from build123d import *

# Parameters (mm, degrees)
SKETCH1_W           = 95
SKETCH1_H           = 95
BOSS_EXTRUDE1_DEPTH = 25
SKETCH2_R           = 7.75
CUT_EXTRUDE2_DEPTH  = 100
SKETCH3_R           = 17
CUT_EXTRUDE3_DEPTH  = 22
CUT_EXTRUDE4_START  = -22
SKETCH4_R           = 17
CUT_EXTRUDE4_DEPTH  = 22
SKETCH5_W           = 6.246993927
SKETCH5_H           = 25
CUT_EXTRUDE5_DEPTH  = 22
SKETCH6_W           = 7.178723585
SKETCH6_H           = 25
CUT_EXTRUDE6_DEPTH  = 22
SKETCH8_W           = 99.503929421
SKETCH8_H           = 3.5
CUT_EXTRUDE7_DEPTH  = 100
SKETCH9_W           = 8.3
SKETCH9_H           = 15.5
CUT_EXTRUDE11_DEPTH = 100
SKETCH13_W          = 87
SKETCH13_H          = 15.5
CUT_EXTRUDE12_DEPTH = 2
SKETCH14_W          = 25.5
SKETCH14_H          = 47
CUT_EXTRUDE14_DEPTH = 18.5
SKETCH16_W          = 24.75
SKETCH16_H          = 47
CUT_EXTRUDE15_DEPTH = 5
SKETCH17_W          = 20.919567191
SKETCH17_H          = 47
CUT_EXTRUDE16_DEPTH = 5
CUT_EXTRUDE17_DEPTH = 100
FILLET6_R           = 1.5
FILLET7_R           = 1.5
FILLET8_R           = 1.5
FILLET9_R           = 1.5
SKETCH19_W          = 12.12120401
SKETCH19_H          = 21.5
CUT_EXTRUDE20_DEPTH = 100
SKETCH20_W          = 5.709228799
SKETCH20_H          = 91
CUT_EXTRUDE23_DEPTH = 100
SKETCH21_W          = 6
SKETCH21_H          = 47
CUT_EXTRUDE26_DEPTH = 40
CHAMFER1_SIZE       = 2
SKETCH22_W          = 15
SKETCH22_H          = 10
CUT_EXTRUDE27_DEPTH = 4
SKETCH23_W          = 2
SKETCH23_H          = 10
CUT_EXTRUDE28_DEPTH = 54
CHAMFER2_SIZE       = 2
CHAMFER3_SIZE       = 4
CHAMFER4_SIZE       = 4
CUT_EXTRUDE29_DEPTH = 100


with BuildPart() as part:
    # Sketch1 → Boss-Extrude1 (new body)
    with BuildSketch(Plane(origin=(0, 0, 0), x_dir=(1, 0, 0), z_dir=(0, 1, 0))):
        with Locations((3.271948822, -17.506298191)):
            Rectangle(SKETCH1_W, SKETCH1_H)
    extrude(amount=BOSS_EXTRUDE1_DEPTH)

    # Sketch2 → Cut-Extrude2 (cut)
    with BuildSketch(Plane.XY.offset(65.006298191)):
        with Locations((-29.228051178, 10.75)):
            Circle(SKETCH2_R)
        with Locations((15.771948822, 10.75)):
            Circle(SKETCH2_R)
    extrude(amount=-CUT_EXTRUDE2_DEPTH, mode=Mode.SUBTRACT)

    # Sketch3 → Cut-Extrude3 (cut)
    with BuildSketch(Plane.XY.offset(65.006298191)):
        with Locations((-29.228051178, 10.75)):
            Circle(SKETCH3_R)
        with Locations((15.771948822, 10.75)):
            Circle(SKETCH3_R)
    extrude(amount=-CUT_EXTRUDE3_DEPTH, mode=Mode.SUBTRACT)

    # Sketch4 → Cut-Extrude4 (cut)
    with BuildSketch(Plane(origin=(0, 0, -29.993701809), x_dir=(-1, 0, 0), z_dir=(0, 0, -1)).offset(CUT_EXTRUDE4_START)):
        with Locations((-15.771948822, 10.75)):
            Circle(SKETCH4_R)
        with Locations((29.228051178, 10.75)):
            Circle(SKETCH4_R)
    extrude(amount=CUT_EXTRUDE4_DEPTH, mode=Mode.SUBTRACT)

    # Sketch5 → Cut-Extrude5 (cut)
    with BuildSketch(Plane.XY.offset(65.006298191)):
        with Locations((-41.104554214, 12.5)):
            Rectangle(SKETCH5_W, SKETCH5_H)
    extrude(amount=-CUT_EXTRUDE5_DEPTH, mode=Mode.SUBTRACT)

    # Sketch6 → Cut-Extrude6 (cut)
    with BuildSketch(Plane(origin=(0, 0, -29.993701809), x_dir=(-1, 0, 0), z_dir=(0, 0, -1))):
        with Locations((40.638689386, 12.5)):
            Rectangle(SKETCH6_W, SKETCH6_H)
    extrude(amount=-CUT_EXTRUDE6_DEPTH, mode=Mode.SUBTRACT)

    # Sketch8 → Cut-Extrude7 (cut)
    with BuildSketch(Plane(origin=(0, 0, -29.993701809), x_dir=(-1, 0, 0), z_dir=(0, 0, -1))):
        with Locations((-1.019984112, 23.25)):
            Rectangle(SKETCH8_W, SKETCH8_H)
    extrude(amount=-CUT_EXTRUDE7_DEPTH, mode=Mode.SUBTRACT)

    # Sketch9 → Cut-Extrude11 (cut)
    with BuildSketch(Plane.XY.offset(65.006298191)):
        with Locations((-7.828051178, 10.75)):
            Rectangle(SKETCH9_W, SKETCH9_H)
    extrude(amount=-CUT_EXTRUDE11_DEPTH, mode=Mode.SUBTRACT)

    # Sketch13 → Cut-Extrude12 (cut)
    with BuildSketch(Plane.ZY.offset(3.678051178)):
        with Locations((17.506298191, 10.75)):
            Rectangle(SKETCH13_W, SKETCH13_H)
    extrude(amount=-CUT_EXTRUDE12_DEPTH, mode=Mode.SUBTRACT)

    # Sketch14 → Cut-Extrude14 (cut)
    with BuildSketch(Plane(origin=(0, 21.5, 0), x_dir=(1, 0, 0), z_dir=(0, 1, 0))):
        with Locations((-6.728051178, -17.506298191)):
            Rectangle(SKETCH14_W, SKETCH14_H)
    extrude(amount=-CUT_EXTRUDE14_DEPTH, mode=Mode.SUBTRACT)

    # Sketch16 → Cut-Extrude15 (cut)
    with BuildSketch(Plane(origin=(0, 21.5, 0), x_dir=(1, 0, 0), z_dir=(0, 1, 0))):
        with Locations((-29.853051178, -17.506298191)):
            Rectangle(SKETCH16_W, SKETCH16_H)
    extrude(amount=-CUT_EXTRUDE15_DEPTH, mode=Mode.SUBTRACT)

    # Sketch17 → Cut-Extrude16 (cut)
    with BuildSketch(Plane(origin=(0, 21.5, 0), x_dir=(1, 0, 0), z_dir=(0, 1, 0))):
        with Locations((16.481732418, -17.506298191)):
            Rectangle(SKETCH17_W, SKETCH17_H)
    extrude(amount=-CUT_EXTRUDE16_DEPTH, mode=Mode.SUBTRACT)

    # Sketch18 → Cut-Extrude17 (cut)
    with BuildSketch(Plane.XY.offset(65.006298191)):
        with BuildLine():
            Line((34.66639245, 12.75), (37.680851122, 12.75))
            ThreePointArc((37.680851122, 12.75), (37.300376381, 15.28065192), (36.628602437, 17.75))
            Line((36.628602437, 17.75), (33.435470555, 17.75))
            ThreePointArc((33.435470555, 17.75), (34.221100776, 15.291893017), (34.66639245, 12.75))
        make_face()
        with BuildLine():
            Line((34.66639245, 8.75), (37.680851122, 8.75))
            ThreePointArc((37.680851122, 8.75), (37.300376381, 6.21934808), (36.628602437, 3.75))
            Line((36.628602437, 3.75), (33.435470555, 3.75))
            ThreePointArc((33.435470555, 3.75), (34.221100776, 6.208106983), (34.66639245, 8.75))
        make_face()
    extrude(amount=-CUT_EXTRUDE17_DEPTH, mode=Mode.SUBTRACT)

    # Fillet6
    fillet6_edges = [part.edges().sort_by_distance(p)[0] for p in [
        (33.435470555, 17.75, 17.506298191),
        (36.628602437, 17.75, 17.506298191),
    ]]
    fillet(fillet6_edges, radius=FILLET6_R - 0.0001)  # a hair under: the kernel refuses the full size

    # Fillet7
    fillet7_edges = [part.edges().sort_by_distance(p)[0] for p in [
        (37.680851122, 12.75, 17.506298191),
        (34.66639245, 12.75, 17.506298191),
    ]]
    fillet(fillet7_edges, radius=FILLET7_R - 0.0001)  # a hair under: the kernel refuses the full size

    # Fillet8
    fillet8_edges = [part.edges().sort_by_distance(p)[0] for p in [
        (33.435470555, 3.75, 17.506298191),
        (36.628602437, 3.75, 17.506298191),
    ]]
    fillet(fillet8_edges, radius=FILLET8_R - 0.0001)  # a hair under: the kernel refuses the full size

    # Fillet9
    fillet9_edges = [part.edges().sort_by_distance(p)[0] for p in [
        (37.680851122, 8.75, 17.506298191),
        (34.66639245, 8.75, 17.506298191),
    ]]
    fillet(fillet9_edges, radius=FILLET9_R - 0.0001)  # a hair under: the kernel refuses the full size

    # Sketch19 → Cut-Extrude20 (cut)
    with BuildSketch(Plane.XY.offset(65.006298191)):
        with Locations((44.711346817, 10.75)):
            Rectangle(SKETCH19_W, SKETCH19_H)
    extrude(amount=-CUT_EXTRUDE20_DEPTH, mode=Mode.SUBTRACT)

    # Sketch20 → Cut-Extrude23 (cut)
    with BuildSketch(Plane(origin=(0, 21.5, 0), x_dir=(1, 0, 0), z_dir=(0, 1, 0))):
        with Locations((35.796130413, -17.506298191)):
            Rectangle(SKETCH20_W, SKETCH20_H)
    extrude(amount=-CUT_EXTRUDE23_DEPTH, mode=Mode.SUBTRACT)

    # Sketch21 → Cut-Extrude26 (cut)
    with BuildSketch(Plane(origin=(0, 21.5, 0), x_dir=(1, 0, 0), z_dir=(0, 1, 0))):
        with Locations((29.941516013, -17.506298191)):
            Rectangle(SKETCH21_W, SKETCH21_H)
    extrude(amount=-CUT_EXTRUDE26_DEPTH, mode=Mode.SUBTRACT)

    # Chamfer1
    chamfer1_edges = [part.edges().sort_by_distance(p)[0] for p in [
        (26.941516013, 16.5, 17.506298191),
    ]]
    chamfer(chamfer1_edges, length=CHAMFER1_SIZE)

    # Sketch22 → Cut-Extrude27 (cut)
    with BuildSketch(Plane(origin=(0, 0, 0), x_dir=(-1, 0, 0), z_dir=(0, -1, 0))):
        with Locations((34.728051178, -17.506298191)):
            Rectangle(SKETCH22_W, SKETCH22_H)
    extrude(amount=-CUT_EXTRUDE27_DEPTH, mode=Mode.SUBTRACT)

    # Sketch23 → Cut-Extrude28 (cut)
    with BuildSketch(Plane(origin=(0, 0, 0), x_dir=(-1, 0, 0), z_dir=(0, -1, 0))):
        with Locations((43.228051178, -17.506298191)):
            Rectangle(SKETCH23_W, SKETCH23_H)
    extrude(amount=-CUT_EXTRUDE28_DEPTH, mode=Mode.SUBTRACT)

    # Chamfer2
    chamfer2_edges = [part.edges().sort_by_distance(p)[0] for p in [
        (-42.228051178, 4, 17.506298191),
    ]]
    chamfer(chamfer2_edges, length=CHAMFER2_SIZE)

    # Chamfer3
    chamfer3_edges = [part.edges().sort_by_distance(p)[0] for p in [
        (-44.228051178, 0, 2.256298191),
    ]]
    chamfer(chamfer3_edges, length=CHAMFER3_SIZE)

    # Chamfer4
    chamfer4_edges = [part.edges().sort_by_distance(p)[0] for p in [
        (-44.228051178, 0, 32.756298191),
    ]]
    chamfer(chamfer4_edges, length=CHAMFER4_SIZE)

    # Sketch24 → Cut-Extrude29 (cut)
    with BuildSketch(Plane.XY.offset(65.006298191)):
        with BuildLine():
            Line((36.983688261, 16.579680704), (37.862836804, 12.677489289))
            ThreePointArc((37.862836804, 12.677489289), (36.729195727, 10.884486805), (34.936193243, 12.018127881))
            Line((34.936193243, 12.018127881), (34.0570447, 15.920319296))
            ThreePointArc((34.0570447, 15.920319296), (35.190685776, 17.713321781), (36.983688261, 16.579680704))
        make_face()
        with BuildLine():
            Line((37.434280479, 6.920319296), (36.555131936, 3.018127881))
            ThreePointArc((36.555131936, 3.018127881), (34.762129451, 1.884486805), (33.628488375, 3.677489289))
            Line((33.628488375, 3.677489289), (34.507636918, 7.579680704))
            ThreePointArc((34.507636918, 7.579680704), (36.300639403, 8.713321781), (37.434280479, 6.920319296))
        make_face()
    extrude(amount=-CUT_EXTRUDE29_DEPTH, mode=Mode.SUBTRACT)


solid = part.part
Can you work these out from the model? Positions are in its coordinate system, mm. A direction names the side the tool comes from. Coordinates: 2 decimals unless noted, no trailing zeros. Order: outer loops, then holes, each group sorted by start corner. A loop starts at its lowest first (then second) coordinate and runs counter-clockwise, first axis right, second up. Notation, with made-up numbers: M -12.75,59 L 33.25,59 A20 ccw 33.25,82 Z; hole C 42.5,35 d11. An arc over 180 degrees is marked long. Answer as CSV lines item,"result".
(1) Suppose I cut it at C-C on x = 30. Please give me the cut outline in (y, z).
Geometry check:
outline,"M 0,-29.99 L 1.45,-29.99 L 1.45,-7.99 L 20.05,-7.99 L 20.05,-29.99 L 21.5,-29.99 L 21.5,-5.99 L 0,-5.99 Z; M 0,41.01 L 21.5,41.01 L 21.5,65.01 L 20.05,65.01 L 20.05,43.01 L 1.45,43.01 L 1.45,65.01 L 0,65.01 Z"
(2) Suppose I cut it at A-A on z = 56. Please give me the cut outline in (x, y), plus the area to 3 significant figures.
Geometry check:
outline,"M -16.06,0 L 2.6,0 A17 cw 2.6,21.5 L -16.06,21.5 A17 cw Z; M 28.94,0 L 32.94,0 L 32.94,21.5 L 28.94,21.5 A17 cw Z; hole M -11.98,3 L -1.68,3 L -1.68,18.5 L -11.98,18.5 Z"
area,"159 mm^2"
(3) On a 3-axis mill with a long thin cutter (end or side, diameter ignored), from which of +Z, -Z, +X, -X, +Y, -Y can I reach the whole of each face in a straight line? I mean faces 1 (the flat face through (34.28, 6.57, -28.98)), 2 (the flat face through (24, 11, -7.994)), 3 (the cylindrical face through (-1.227, 10.913, 54.16)), 4 (the flat face through (32.942, 11, 52)). Say none if no direction works.
Geometry check:
face 1,"+Z, -Z"
face 2,"-Z"
face 3,"+Z"
face 4,"+X, +Y, -Y"
(4) Please list where these lines run through material, in increasing order: L1, parallel to Z at x = 19.5, y = 20.5; L2, parallel to Y at x = -3.5, z = 51.5; L3, parallel to X at y = 9.75, z = -7.5.
Geometry check:
L1,"-7.99 to -5.99, 41.01 to 43.01"
L2,"0 to 3, 18.5 to 21.5"
L3,"-44.23 to -36.91, -21.54 to -11.98, -1.68 to 8.09, 23.46 to 32.94"
(5) Suppose I cut it at B-B on z = 28. Please give me the cut outline in (x, y).
Geometry check:
outline,"M -44.23,4 L -40.23,0 L 26.94,0 L 26.94,14.5 L 24.94,16.5 L 20.97,16.5 A7.75 cw long 10.58,16.5 L 6.02,16.5 L 6.02,3 L -19.48,3 L -19.48,16.5 L -24.03,16.5 A7.75 cw long -34.42,16.5 L -42.23,16.5 L -42.23,21.5 L -44.23,21.5 Z"
(6) If we mould it in two halves opening along Y, with no side actions, what happens to faces 5 (the cylindrical face through (-35.378, 6.034, 17.863)), 6 (the flat face through (-42.26, 2.03, 32.9)), 7 (the flat face through (38.651, 11, -29))? For each: released by +Y, released by -Y, zero draft, split by the parting line, or undercut.
Geometry check:
face 5,"undercut"
face 6,"released by -Y"
face 7,"zero draft"
(7) I'm going to push flat-ended pins straight in: pin 1 (5 mm diameter, centred on y = 7, z = 16, fed in from -X); pin 2 (10 mm diameter, centred on y = 19, z = 16, fed in from -X); pin 3 (11 mm diameter, centred on x = 6.5, y = 5.5, fed in from +Z); pin 4 (4.5 mm diameter, centred on x = 23, z = 26, fed in from +Y). Where does each tip first touch, or does it pass through?
Geometry check:
pin 1,"x = -42.23"
pin 2,"x = -44.23"
pin 3,"z = 43.01"
pin 4,"y = 16.5"
(8) Suppose I cut it at D-D on x = 0. Please give me the cut outline in (y, z).
Geometry check:
outline,"M 0,-29.99 L 4.41,-29.99 L 4.41,-7.99 L 17.09,-7.99 L 17.09,-29.99 L 21.5,-29.99 L 21.5,-5.99 L 3,-5.99 L 3,41.01 L 21.5,41.01 L 21.5,65.01 L 17.09,65.01 L 17.09,43.01 L 4.41,43.01 L 4.41,65.01 L 0,65.01 Z"
